```python
from build123d import *

# Parameters (mm, degrees)
F1_DEPTH = 101.6


with BuildPart() as f1:
    # F0 (on Top) → F1 (new body)
    with BuildSketch(Plane.XY):
        Polygon((-38.758028, -104.798459), (110.137142, 18.833792), (-71.379113, 85.964666), (-69.320055, 73.923605), (-40.099562, -96.953376), align=None)
        Polygon((-61.59973, 73.923605), (94.819585, 16.385128), (-33.219855, -90.308734), align=None, mode=Mode.SUBTRACT)
        with BuildLine():
            ThreePointArc((-71.379113, 85.964666), (-133.798783, -22.880006), (-38.758028, -104.798459))
            Line((-38.758028, -104.798459), (-40.099562, -96.953376))
            ThreePointArc((-40.099562, -96.953376), (-125.023249, -23.538701), (-69.320055, 73.923605))
            Line((-69.320055, 73.923605), (-71.379113, 85.964666))
        make_face()
    extrude(amount=F1_DEPTH)


solid = f1.part
```
Verification items for the finished model (mm, model axes). A direction names the side the tool comes from. Give positions to 0.01 mm unless a question says otherwise; leave off trailing zeros. Loops run counter-clockwise (first coordinate to the right, second up) from the corner with the lowest first, then second, coordinate; pieces in that order, holes last. Notation, with made-up numbers: M -32,20 L -2,20 A29 ccw -2,48 Z; hole C 9,66.5 d8. An arc over 180 degrees is marked long. Return JSON: item names as keys, results as strings.
1) Tool access check on faces 1 (the flat face through (31.7, -36.21, 50.09)), 2 (the cylindrical face through (-134.1, -21, 50.1)). Record the directions out of +Z, -Z, +X, -X, +Y, -Y that give a thin tool (end or side, any length) a straight path to the whole face; none if there is none.
Findings:
{"face 1": "+Z, -Z", "face 2": "+Z, -Z, -X"}
2) Section check C-C, the plane x = 78.5. Enter the section's corners in (y, z), and give its area (3 significant figures).
Findings:
{"outline": "M -7.44,0 L 2.79,0 L 2.79,101.6 L -7.44,101.6 Z; M 22.39,0 L 30.53,0 L 30.53,101.6 L 22.39,101.6 Z", "area": "1,870 mm2"}
3) Section check A-A, the plane z = 23.5. Enter the section's corners in (x, y), and give its area (3 significant figures).
Findings:
{"outline": "M -71.38,85.96 A98.55 ccw -38.76,-104.8 L 110.14,18.83 Z; hole M -69.32,73.92 A88.33 ccw -40.1,-96.95 Z; hole M -61.6,73.92 L -33.22,-90.31 L 94.82,16.39 Z", "area": "6,520 mm2"}
4) Gauge pin test, flat ends, axial feed: P1, Ø6, axis at y = -14.5, z = 80, coming from the -X side; P2, Ø3, axis at x = -69, z = 51.5, coming from the +Y side; P3, Ø4, axis at y = -20, z = 91, coming from the +X side. Record the tip position at first contact, or that the pin passes through.
Findings:
{"P1": "stops at x = -135.07", "P2": "stops at y = 85.64", "P3": "stops at x = 65.78"}
5) Section check D-D, the plane x = -54.5. Enter the section's corners in (y, z), and give its area (3 significant figures).
Findings:
{"outline": "M -103.19,0 L -95.42,0 L -95.42,101.6 L -103.19,101.6 Z; M -12.74,0 L 32.84,0 L 32.84,101.6 L -12.74,101.6 Z; M 71.31,0 L 79.72,0 L 79.72,101.6 L 71.31,101.6 Z", "area": "6,280 mm2"}
6) Material ranges on L1, parallel to X at y = 5, z = 9; L2, parallel to X at y = -3, z = 23; L3, parallel to Y at x = -111, z = 93, recorded low to high. Write a range as [from, to].
Findings:
{"L1": "x = [-134.56, -125.23], [-57.53, -49.69], [81.16, 93.48]", "L2": "x = [-135.15, -126.11], [-56.17, -48.31], [71.56, 83.84]", "L3": "y = [-70.96, -58.32], [41.02, 58.43]"}
7) Section check B-B, the plane y = 41. Enter the section's corners in (x, z).
Findings:
{"outline": "M -123.13,0 L -111.01,0 L -111.01,101.6 L -123.13,101.6 Z; M -63.69,0 L -55.91,0 L -55.91,101.6 L -63.69,101.6 Z; M 27.9,0 L 50.2,0 L 50.2,101.6 L 27.9,101.6 Z"}
